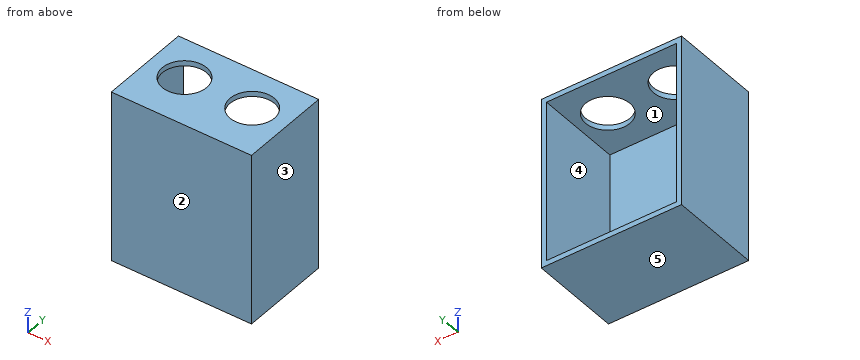
Solid Edge part; units mm, degrees
sketch "Sketch1" plane through (0, 0, 0) normal (0, 0, 1) x (1, 0, 0)
  line L0 (-23.7696, -8.3107) -> (22.0304, -8.3107)
  line L1 (22.0304, -8.3107) -> (22.0304, 13.1893)
  line L2 (22.0304, 13.1893) -> (-23.7696, 13.1893)
  line L3 (-23.7696, 13.1893) -> (-23.7696, -8.3107)
extrude "Protrusion1" add sketch "Sketch1" along normal blind 2
sketch "Sketch2" plane through (-0.8696, 2.4393, 2) normal (0, 0, 1) x (1, 0, 0)
  circle A0 centre (-13, 0) radius 8.5
  circle A1 centre (13, 0) radius 8.5
extrude "ExtrudedCutout_1" cut sketch "Sketch2" against normal blind 110.6455
sketch "Sketch3" plane through (-0.8696, 2.4393, 2) normal (0, 0, 1) x (1, 0, 0)
  line L0 (-22.9, 10.75) -> (-24.9, 10.75)
  line L1 (-24.9, 10.75) -> (-24.9, -10.75)
  line L2 (-24.9, -10.75) -> (-22.9, -10.75)
  line L3 (-22.9, -10.75) -> (-22.9, 10.75)
  line L4 (22.9, 10.75) -> (24.9, 10.75)
  line L5 (24.9, 10.75) -> (24.9, -10.75)
  line L6 (24.9, -10.75) -> (22.9, -10.75)
  line L7 (22.9, -10.75) -> (22.9, 10.75)
extrude "ExtrudedProtrusion_2" add sketch "Sketch3" against normal blind 2
sketch "Sketch4" plane through (-0.8696, 2.4393, 2) normal (0, 0, 1) x (1, 0, 0)
  line L0 (-24.9, 10.75) -> (-26.9, 10.75)
  line L1 (-26.9, 10.75) -> (-26.9, -10.75)
  line L2 (-26.9, -10.75) -> (-24.9, -10.75)
  line L3 (-24.9, -10.75) -> (-24.9, 10.75)
  line L4 (24.9, 10.75) -> (26.9, 10.75)
  line L5 (26.9, 10.75) -> (26.9, -10.75)
  line L6 (26.9, -10.75) -> (24.9, -10.75)
  line L7 (24.9, -10.75) -> (24.9, 10.75)
extrude "ExtrudedProtrusion_4" add sketch "Sketch4" against normal blind 66
sketch "Sketch5" plane through (24.0304, 2.4393, -32) normal (-1, 0, 0) x (0, 0, 1)
  line L0 (-32, 10.75) -> (-30, 10.75)
  line L1 (-30, 10.75) -> (-30, -10.75)
  line L2 (-30, -10.75) -> (-32, -10.75)
  line L3 (-32, -10.75) -> (-32, 10.75)
extrude "ExtrudedProtrusion_5" add sketch "Sketch5" along normal blind 49.8416
sketch "Sketch6" plane through (-0.8696, -8.3107, -31) normal (0, -1, 0) x (-1, 0, 0)
  line L0 (-26.9, 33) -> (26.9, 33)
  line L1 (26.9, 33) -> (26.9, -32.0416)
  line L2 (26.9, -33) -> (26.9, -32.0416)
  line L3 (-26.9, -33) -> (26.9, -33)
  line L4 (-26.9, -33) -> (-26.9, 33)
extrude "ExtrudedProtrusion_6" add sketch "Sketch6" along normal blind 8.5
sketch "Sketch7" plane through (-0.8696, -8.3107, -31) normal (0, 1, 0) x (1, 0, 0)
  line L0 (-24.9, 31) -> (24.9, 31)
  line L1 (24.9, 31) -> (24.9, -31)
  line L2 (24.9, -31) -> (-24.9, -31)
  line L3 (-24.9, -31) -> (-24.9, 31)
extrude "ExtrudedCutout_2" cut sketch "Sketch7" against normal blind 6.5
sketch "Sketch8" plane through (-0.8696, 13.1893, -31) normal (0, 1, 0) x (0, 0, 1)
  line L0 (-33, 26.9) -> (33, 26.9)
  line L1 (33, 26.9) -> (33, -26.9)
  line L2 (33, -26.9) -> (-33, -26.9)
  line L3 (-33, -26.9) -> (-33, 26.9)
extrude "ExtrudedProtrusion_7" add sketch "Sketch8" along normal blind 5
sketch "Sketch9" plane through (-0.8696, 18.1893, -31) normal (0, 1, 0) x (0, 0, 1)
  line L0 (-31, 24.9) -> (31, 24.9)
  line L1 (31, 24.9) -> (31, -24.9)
  line L2 (31, -24.9) -> (-31, -24.9)
  line L3 (-31, -24.9) -> (-31, 24.9)
extrude "ExtrudedCutout_3" cut sketch "Sketch9" against normal blind 33
Could you check a few things on this model? Use its own coordinates, in mm. Face numbers are marked on the shaded views. A direction names the side the tool comes from. Give positions to 0.01 mm unless a question says otherwise; leave off trailing zeros. Write each loop counter-clockwise with the first axis right and the second up, starting at its lowest first coordinate (ties: lowest second). Pieces come first, ordered by that corner, then holes. Notation, with made-up numbers: (76, 9.5) - (106, 9.5) arc R9 cw to (106, 15.5) - close; hole circle Ø7 at (-18, 21.25). An arc over 180 degrees is marked (long way). One line per item, written item: value. Start each with the question number.
Item 1: Which directions (+Z, -Z, +X, -X, +Y, -Y) give clear straight access to the entire face, cutting with the end or side of a thin tool? Please do the marked faces 1 and 2.
Item 2: Imagine slicing it at B-B, the plane y = -4.5. List the corners of the cut face in (x, z) for me, and give its area (3 significant figures).
Item 3: Imagine slicing it at D-D, the plane z = -41. List the corners of the cut face in (x, y) for me.
Item 4: Imagine slicing it at A-A, the plane x = -18. List the corners of the cut face in (y, z) for me.
Item 5: If we mould it in two halves opening along Z, with no side actions, what happens to the marked faces 3, 4 and 5? For each: +Z half, -Z half, draft (parallel to the pull), parting line (faces both ways), or undercut.
Item 6: Please list where these lines run through material, in increasing order: line 1 (Z direction, x = -21.5, y = -9.5); line 2 (X direction, y = 6, z = -14); line 3 (Y direction, x = 18.5, z = -14). Write a range as from..to.
Item 7: Imagine slicing it at C-C, the plane y = 12.5. List the corners of the cut face in (x, z) for me, and give its area (3 significant figures).
Item 8: I'm going to push flat-ended pins straight in: pin 1 (10 mm diameter, centred on x = -10.5, y = 3, fed in from +Z); pin 2 (4 mm diameter, centred on x = -7.5, z = -31.5, fed in from +Y). Where does each tip first touch, or does it pass through?
Geometry says:
1. face 1: +Y
1. face 2: +Z, -Z, +X, -X, -Y
2. outline: (-27.77, -64) - (26.03, -64) - (26.03, 2) - (17.04, 2) - (17.04, 0) - (24.03, 0) - (24.03, -62) - (-25.77, -62) - (-25.77, 0) - (-18.78, 0) - (-18.78, 2) - (-27.77, 2) - close; (-8.96, 0) - (7.22, 0) - (7.22, 2) - (-8.96, 2) - close
2. area: 424 mm^2
3. outline: (-27.77, -16.81) - (26.03, -16.81) - (26.03, 18.19) - (24.03, 18.19) - (24.03, -14.81) - (-25.77, -14.81) - (-25.77, 18.19) - (-27.77, 18.19) - close
4. outline: (-16.81, -64) - (18.19, -64) - (18.19, -62) - (-14.81, -62) - (-14.81, 0) - (-4.99, 0) - (-4.99, 2) - (-16.81, 2) - close; (9.87, 0) - (18.19, 0) - (18.19, 2) - (9.87, 2) - close
5. face 3: draft
5. face 4: undercut
5. face 5: -Z half
6. line 1: -64..-62, 0..2
6. line 2: -27.77..-25.77, 24.03..26.03
6. line 3: -16.81..-14.81
7. outline: (-27.77, -64) - (26.03, -64) - (26.03, 2) - (-27.77, 2) - close; hole (-25.77, -62) - (24.03, -62) - (24.03, 0) - (-25.77, 0) - close
7. area: 463 mm^2
8. pin 1: z = -62
8. pin 2: y = -14.81
